Design review of the part built by this model. Coordinates are the model's own, in mm. Face numbers are marked on the shaded views. A direction names the side the tool comes from. Give positions to 0.01 mm unless a question says otherwise; leave off trailing zeros. Order: outer loops, then holes, each group sorted by start corner. A loop starts at its lowest first (then second) coordinate and runs counter-clockwise, first axis right, second up.
```python
from build123d import *

# Parameters (mm, degrees)
F0_W     = 229.52804
F0_H     = 152.525924
F1_DEPTH = 6.35
F2_W     = 23.711868
F2_H     = 24.674061
F3_DEPTH = 155.448
F4_W     = 25.340267
F4_H     = 24.805527
F5_DEPTH = 155.448
F6_W     = 27.706921
F6_H     = 27.038488
F6_W_2   = 24.087668
F6_H_2   = 23.228791
F7_DEPTH = 155.448


with BuildPart() as f1:
    # F0 (on Top) → F1 (new body)
    with BuildSketch(Plane.XY):
        with Locations((8.701302, -4.533436)):
            Rectangle(F0_W, F0_H)
    extrude(amount=F1_DEPTH)

    # F2 (on face) → F3 (join)
    with BuildSketch(Plane.XY.offset(6.35)):
        with Locations((111.609388, -68.459367)):
            Rectangle(F2_W, F2_H)
    extrude(amount=F3_DEPTH)

    # F4 (on face) → F5 (join)
    with BuildSketch(Plane.XY.offset(6.35)):
        with Locations((110.795188, 59.326762)):
            Rectangle(F4_W, F4_H)
    extrude(amount=F5_DEPTH)

    # F6 (on face) → F7 (join)
    with BuildSketch(Plane.XY.offset(6.35)):
        with Locations((-92.209257, -67.277154)):
            Rectangle(F6_W, F6_H)
        with Locations((-94.018884, 60.11513)):
            Rectangle(F6_W_2, F6_H_2)
    extrude(amount=F7_DEPTH)


solid = f1.part
```
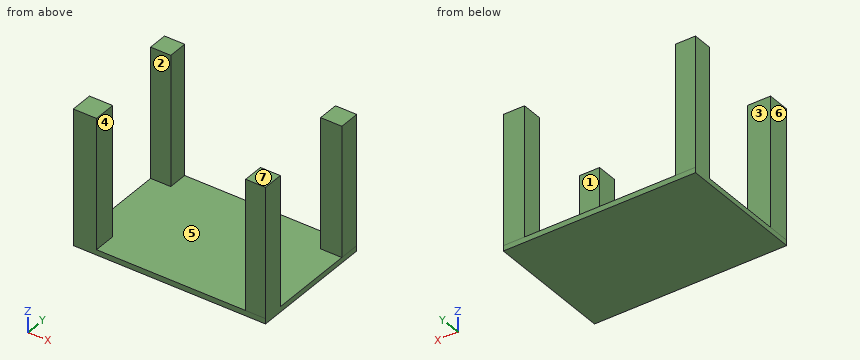
1. Machinability: for the marked faces 1, 2 and 3, which of the approach directions +Z, -Z, +X, -X, +Y, -Y give a long, thin tool a straight path to every point of the face, cutting with its end or side? Answer none if there is none.
Recorded:
face 1: +Z, +X
face 2: +Z, -X
face 3: +Z, +X, -X
2. For line 1 along X through (y, z) = (-63.5, 121); line 2 along X through (y, z) = (50.5, 113.5); line 3 along Z through (x, y) = (-46.5, 3.5), list the stretches that pass through material, from the lowest coordinate up.
Recorded:
line 1: x = -106.06 to -78.36, 99.75 to 123.47
line 2: x = -106.06 to -81.98, 98.13 to 123.47
line 3: z = 0 to 6.35
3. Draft analysis for pull direction X (two halves, no side actions). For the marked faces 4, 5, 6 and 7, state which applies: pulls with the +X half, pulls with the -X half, needs draft (parallel to the pull), parting line crosses it, or undercut.
Recorded:
face 4: undercut
face 5: undercut
face 6: pulls with the -X half
face 7: needs draft
4. Take a section at A-A (z = 126.5). State the section outline as (x, y) points.
Recorded:
outline: (-106.06, -80.8) - (-78.36, -80.8) - (-78.36, -53.76) - (-106.06, -53.76) - close; (-106.06, 48.5) - (-81.98, 48.5) - (-81.98, 71.73) - (-106.06, 71.73) - close; (98.13, 46.92) - (123.47, 46.92) - (123.47, 71.73) - (98.13, 71.73) - close; (99.75, -80.8) - (123.47, -80.8) - (123.47, -56.12) - (99.75, -56.12) - close
5. Take a section at D-D (y = 8). State the section outline as (x, z) points.
Recorded:
outline: (-106.06, 0) - (123.47, 0) - (123.47, 6.35) - (-106.06, 6.35) - close
6. Take a section at B-B (y = 58.5). State the section outline as (x, z) points, then the cut area to 3 significant figures.
Recorded:
outline: (-106.06, 0) - (123.47, 0) - (123.47, 161.8) - (98.13, 161.8) - (98.13, 6.35) - (-81.98, 6.35) - (-81.98, 161.8) - (-106.06, 161.8) - close
area: 9,140 mm2
7. Take a section at C-C (x = -61.5). State the section outline as (y, z) points, then the cut area to 3 significant figures.
Recorded:
outline: (-80.8, 0) - (71.73, 0) - (71.73, 6.35) - (-80.8, 6.35) - close
area: 969 mm2
8. For pin 1 (3 mm diameter, centred on x = 12, y = -46.5, fed in from +Z), flat-tipped, find the tip position at first contact; note if it passes through.
Recorded:
pin 1: stops at z = 6.35
